from build123d import *

# Parameters (mm, degrees)
CHAMFER1_SIZE = 1.27
FILLET1_R     = 7.62


with BuildPart() as part:
    # Sketch1 → Revolve1 (revolve)
    with BuildSketch(Plane.XY, mode=Mode.PRIVATE) as revolve1_sk:
        Polygon((0, 28.575), (0, 35.71875), (12.7, 35.71875), (12.7, 39.6621), (25.4, 39.6621), (25.4, 28.575), align=None)
    revolve(revolve1_sk.sketch.rotate(Axis((-88.99, 0, 0), (1, 0, 0)), 90), axis=Axis((-88.99, 0, 0), (1, 0, 0)))

    # Chamfer1
    chamfer1_edges = [part.edges().sort_by_distance(p)[0] for p in [
        (25.4, 0, -39.6621),
        (12.7, 0, -39.6621),
        (0, 0, -35.71875),
        (0, 0, -28.575),
    ]]
    chamfer(chamfer1_edges, length=CHAMFER1_SIZE)

    # Fillet1
    fillet1_edges = [part.edges().sort_by_distance(p)[0] for p in [
        (25.4, 0, -28.575),
    ]]
    fillet(fillet1_edges, radius=FILLET1_R)


solid = part.part
Source: CAD feature listing. Evaluate the final solid. Frame: model axes, mm. Round coordinates to 2 decimals unless told otherwise and drop trailing zeros. Write each loop counter-clockwise with the first axis right and the second up, starting at its lowest first coordinate (ties: lowest second). Pieces come first, ordered by that corner, then holes. Notation, with made-up numbers: M 45,24 L 65,24 A9 cw 65,39 Z; hole C 67,-19 d1. An arc over 180 degrees is marked long. One line per item, written item: value. Start each with the question number.
Item 1: Pin query (flat end, axial travel): pin 1 (12 mm diameter, centred on x = 3.5, z = 0.5, fed in from +Y); pin 2 (5 mm diameter, centred on y = 9.5, z = -29.5, fed in from +X). Return the tip coordinate at first contact, or that it passes through.
Item 2: Mould query, pull axis Z, two halves, no side actions, for faces 1 (the cylindrical face through (9.409, -1.256, -28.547)), 2 (the cylindrical face through (7.07, -30.12, 19.2)), 3 (the flat face through (12.7, 25.4, -25.4)). Classes: pulls with the +Z half, pulls with the -Z half, needs draft (parallel to the pull), parting line crosses it, or undercut.
Item 3: Section query D-D (x = 21). Return the cut outline in (y, z).
Item 4: Section query A-A (z = 0). Return the cut outline in (x, y) (3 decimals).
Item 5: Ray query, L1, parallel to Y at x = 3.25, z = -1; L2, parallel to Z at x = 1.5, y = -14; L3, parallel to Y at x = 13.5, z = -12.5. Return the intervals inside material, ascending. Write a range as from..to.
Result set:
1. pin 1: stops at y = 35.72
1. pin 2: stops at x = 24.9
2. face 1: undercut
2. face 2: parting line crosses it
2. face 3: needs draft
3. outline: C 0,0 d79.32; hole C 0,0 d58.58
4. outline: M 0,-34.449 L 1.27,-35.719 L 12.7,-35.719 L 12.7,-38.392 L 13.97,-39.662 L 24.13,-39.662 L 25.4,-38.392 L 25.4,-36.195 A7.62 ccw 17.78,-28.575 L 1.27,-28.575 L 0,-29.845 Z; M 0,29.845 L 1.27,28.575 L 17.78,28.575 A7.62 ccw 25.4,36.195 L 25.4,38.392 L 24.13,39.662 L 13.97,39.662 L 12.7,38.392 L 12.7,35.719 L 1.27,35.719 L 0,34.449 Z
5. L1: y = -35.7..-28.56, 28.56..35.7
5. L2: z = -32.86..-24.91, 24.91..32.86
5. L3: y = -37.15..-25.7, 25.7..37.15
